The listing builds one solid part. Answer for the finished solid, in the listing's coordinates (mm). Face numbers are marked on the shaded views. A direction names the side the tool comes from. Round coordinates to 2 decimals unless told otherwise and drop trailing zeros. Write each loop counter-clockwise with the first axis right and the second up, starting at its lowest first coordinate (ties: lowest second). Pieces come first, ordered by that corner, then holes. Notation, with made-up numbers: (79.25, 16) - (117.25, 16) arc R23 ccw to (117.25, 44) - close; hole circle Ø4 at (41, -28). An arc over 180 degrees is marked (long way). Answer in a Markdown table with one row per item.
from build123d import *

# Parameters (mm, degrees)
SKETCH_1_W          = 41.5
SKETCH_1_H          = 40
EXTRUDE_1_DEPTH     = 1.5
SKETCH_2_W          = 1.5
SKETCH_2_H          = 40
EXTRUDE_2_DEPTH     = 44.6
FILLET_2_R          = 20
FILLET_3_R          = 20
SKETCH_3_R          = 1.25
SKETCH_3_R_2        = 6
CUT_EXTRUDE_1_DEPTH = 44.6
SKETCH_4_R          = 1.65
CUT_EXTRUDE_2_DEPTH = 44.6
FILLET_5_R          = 2
FILLET_6_R          = 2
FILLET_7_R          = 1.5


with BuildPart() as part:
    # Эскиз1 → Бобышка-Вытянуть1 (new body)
    with BuildSketch(Plane(origin=(0, 0, 0), x_dir=(1, 0, 0), z_dir=(0, 1, 0))):
        Rectangle(SKETCH_1_W, SKETCH_1_H)
    extrude(amount=EXTRUDE_1_DEPTH)

    # Эскиз2 → Бобышка-Вытянуть2 (add)
    with BuildSketch(Plane(origin=(0, 1.5, 0), x_dir=(1, 0, 0), z_dir=(0, 1, 0))):
        with Locations((-20, 0)):
            Rectangle(SKETCH_2_W, SKETCH_2_H)
    extrude(amount=EXTRUDE_2_DEPTH)

    # Скругление2
    fillet_2_edges = [part.edges().sort_by_distance(p)[0] for p in [
        (-20, 46.1, 20),
    ]]
    fillet(fillet_2_edges, radius=FILLET_2_R)

    # Скругление3
    fillet_3_edges = [part.edges().sort_by_distance(p)[0] for p in [
        (-20, 46.1, -20),
    ]]
    fillet(fillet_3_edges, radius=FILLET_3_R - 0.0001)  # a hair under: the kernel refuses the full size

    # Эскиз3 → Вырез-Вытянуть1 (cut)
    with BuildSketch(Plane.ZY.offset(20.75)):
        with Locations((-15.5, 26.1)):
            Circle(SKETCH_3_R)
        with Locations((-7.75, 39.523393759)):
            Circle(SKETCH_3_R)
        with Locations((7.75, 39.523393759)):
            Circle(SKETCH_3_R)
        with Locations((15.5, 26.1)):
            Circle(SKETCH_3_R)
        with Locations((7.75, 12.676606241)):
            Circle(SKETCH_3_R)
        with Locations((-7.75, 12.676606241)):
            Circle(SKETCH_3_R)
        with Locations((0, 19.1)):
            Circle(SKETCH_3_R_2)
    extrude(amount=-CUT_EXTRUDE_1_DEPTH, mode=Mode.SUBTRACT)

    # Эскиз4 → Вырез-Вытянуть2 (cut)
    with BuildSketch(Plane.XZ):
        with Locations(Location((12.75, 15, 0), (0, 0, 270))):
            Circle(SKETCH_4_R)
        with Locations(Location((-10.75, 15, 0), (0, 0, 270))):
            Circle(SKETCH_4_R)
        with Locations(Location((-10.75, -15, 0), (0, 0, 270))):
            Circle(SKETCH_4_R)
        with Locations(Location((12.75, -15, 0), (0, 0, 270))):
            Circle(SKETCH_4_R)
    extrude(amount=-CUT_EXTRUDE_2_DEPTH, mode=Mode.SUBTRACT)

    # Скругление5
    fillet_5_edges = [part.edges().sort_by_distance(p)[0] for p in [
        (20.75, 0.75, -20),
        (20.75, 0.75, 20),
    ]]
    fillet(fillet_5_edges, radius=FILLET_5_R)

    # Скругление6
    fillet_6_edges = [part.edges().sort_by_distance(p)[0] for p in [
        (-20.75, 0, 0),
    ]]
    fillet(fillet_6_edges, radius=FILLET_6_R)

    # Скругление7
    fillet_7_edges = [part.edges().sort_by_distance(p)[0] for p in [
        (-19.25, 1.5, 0),
    ]]
    fillet(fillet_7_edges, radius=FILLET_7_R)


solid = part.part
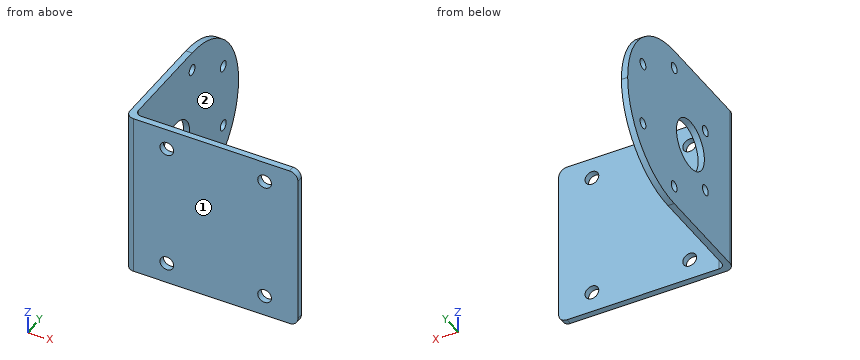
(1) Find the intervals of material crossed by line 1 (Y direction, x = -19.65, z = -7.75); line 2 (Y direction, x = -20, z = 7) (3 decimals); line 3 (X direction, y = 39, z = -13), in increasing order.
Checked values:
| item | result |
|---|---|
| line 1 | y = 0.21 to 11.43, 13.93 to 38.27, 40.77 to 44.54 |
| line 2 | y = 0.439 to 11.677, 13.677 to 38.523, 40.523 to 44.835 |
| line 3 | x = -20.75 to -19.25 |
(2) Section A-A (x = -10.75) is taken. Give the vertices of the cut face in (y, z), and give its area (3 significant figures).
Checked values:
| item | result |
|---|---|
| outline | (0, -20) - (1.5, -20) - (1.5, -16.65) - (0, -16.65) - close; (0, -13.35) - (1.5, -13.35) - (1.5, 13.35) - (0, 13.35) - close; (0, 16.65) - (1.5, 16.65) - (1.5, 20) - (0, 20) - close |
| area | 50.1 mm2 |
(3) Section B-B (y = 19.1) is taken. Give the vertices of the cut face in (x, z), and give its area (3 significant figures).
Checked values:
| item | result |
|---|---|
| outline | (-20.75, -20) - (-19.25, -20) - (-19.25, -6) - (-20.75, -6) - close; (-20.75, 6) - (-19.25, 6) - (-19.25, 20) - (-20.75, 20) - close |
| area | 42.0 mm2 |
(4) Section C-C (z = 12) is taken. Give the vertices of the cut face in (x, y).
Checked values:
| item | result |
|---|---|
| outline | (-20.75, 2) arc R2 ccw to (-18.75, 0) - (20.75, 0) - (20.75, 1.5) - (-17.75, 1.5) arc R1.5 cw to (-19.25, 3) - (-19.25, 42.1) - (-20.75, 42.1) - close |
(5) Flat-ended cylindrical pins translate along their axes: pin 1 (1 mm diameter, centred on y = 19, z = 13, fed in from +X); pin 2 (2 mm diameter, centred on y = 12.68, z = 7.75, fed in from -X); pin 3 (1.5 mm diameter, centred on x = 5, z = -2, fed in from +Y); pin 4 (10 mm diameter, centred on x = -3, z = 11.5, fed in from -Y). Find the tip coordinate at first contact, or state that the pin passes through.
Checked values:
| item | result |
|---|---|
| pin 1 | stops at x = -19.25 |
| pin 2 | passes through |
| pin 3 | stops at y = 1.5 |
| pin 4 | stops at y = 0 |
(6) Section D-D (z = -16) is taken. Give the vertices of the cut face in (x, y), and give its area (3 significant figures).
Checked values:
| item | result |
|---|---|
| outline | (-20.75, 2) arc R2 ccw to (-18.75, 0) - (-12.06, 0) - (-12.06, 1.5) - (-17.75, 1.5) arc R1.5 cw to (-19.25, 3) - (-19.25, 24.95) - (-20.75, 24.95) - close; (-20.75, 27.25) - (-19.25, 27.25) - (-19.25, 38.1) - (-20.75, 38.1) - close; (-9.44, 0) - (11.44, 0) - (11.44, 1.5) - (-9.44, 1.5) - close; (14.06, 0) - (20.75, 0) - (20.75, 1.5) - (14.06, 1.5) - close |
| area | 105 mm2 |
(7) For the marked faces 1 and 2, determine the directions among +Z, -Z, +X, -X, +Y, -Y from which every point of the face is accessible in a straight line to the end or side of a thin tool.
Checked values:
| item | result |
|---|---|
| face 1 | +Z, -Z, +X, -X, -Y |
| face 2 | +Z, -Z, +X, +Y |
